from build123d import *

# Parameters (mm, degrees)
F2_DEPTH = 1
F3_W     = 90
F3_H     = 3.5
F3_H_2   = 0.0419686139
F3_H_3   = 3.4580313861
F4_DEPTH = 2
F5_W     = 90
F5_H     = 3.5
F5_H_2   = 4.5
F5_H_3   = 8.0419686139
F6_DEPTH = 1


# Not quite as in the source:
# - a feature names something its author has since deleted; it is built from what else it names


with BuildPart() as f2:
    # F1 (on face) → F2 (new body)
    with BuildSketch(Plane.XY):
        with BuildLine():
            Line((14.8598281033, 4.21106866), (-75.1401718967, 4.21106866))
            Line((-75.1401718967, 4.21106866), (-75.1401718967, 0.21106866))
            Line((-75.1401718967, 0.21106866), (4.3706398308, 0.21106866))
            ThreePointArc((4.3706398308, 0.21106866), (5.7848533932, -0.3747177776), (6.3706398308, -1.78893134))
            Line((6.3706398308, -1.78893134), (6.3706398308, -3.78893134))
            Line((6.3706398308, -3.78893134), (14.8598281033, -3.78893134))
            Line((14.8598281033, -3.78893134), (14.8598281033, 4.21106866))
        make_face()
        with BuildLine():
            Line((14.8598281033, -49.78893134), (6.3706398308, -49.78893134))
            Line((6.3706398308, -49.78893134), (6.3706398308, -51.78893134))
            ThreePointArc((6.3706398308, -51.78893134), (5.7848533932, -53.2031449024), (4.3706398308, -53.78893134))
            Line((4.3706398308, -53.78893134), (-75.1401718967, -53.78893134))
            Line((-75.1401718967, -53.78893134), (-75.1401718967, -57.78893134))
            Line((-75.1401718967, -57.78893134), (14.8598281033, -57.78893134))
            Line((14.8598281033, -57.78893134), (14.8598281033, -49.78893134))
        make_face()
        with BuildLine():
            Line((-75.1401718967, -3.78893134), (-75.1401718967, 0.21106866))
            Line((-75.1401718967, 0.21106866), (-77.6293601692, 0.21106866))
            ThreePointArc((-77.6293601692, 0.21106866), (-79.0435737315, -0.3747177776), (-79.6293601692, -1.78893134))
            Line((-79.6293601692, -1.78893134), (-79.6293601692, -51.78893134))
            ThreePointArc((-79.6293601692, -51.78893134), (-79.0435737315, -53.2031449024), (-77.6293601692, -53.78893134))
            Line((-77.6293601692, -53.78893134), (-75.1401718967, -53.78893134))
            Line((-75.1401718967, -53.78893134), (-75.1401718967, -49.78893134))
            Line((-75.1401718967, -49.78893134), (-75.1401718967, -3.78893134))
        make_face()
        with BuildLine():
            Line((-68.8141618371, -49.78893134), (-75.1401718967, -49.78893134))
            Line((-75.1401718967, -49.78893134), (-75.1401718967, -53.78893134))
            Line((-75.1401718967, -53.78893134), (4.3706398308, -53.78893134))
            ThreePointArc((4.3706398308, -53.78893134), (5.7848533932, -53.2031449024), (6.3706398308, -51.78893134))
            Line((6.3706398308, -51.78893134), (6.3706398308, -49.78893134))
            Line((6.3706398308, -49.78893134), (6.1858381629, -49.78893134))
            Line((6.1858381629, -49.78893134), (0.4592296318, -49.78893134))
            Line((0.4592296318, -49.78893134), (-68.8141618371, -49.78893134))
        make_face()
        with BuildLine():
            Line((4.3706398308, 0.21106866), (-75.1401718967, 0.21106866))
            Line((-75.1401718967, 0.21106866), (-75.1401718967, -3.78893134))
            Line((-75.1401718967, -3.78893134), (-68.8141618371, -3.78893134))
            Line((-68.8141618371, -3.78893134), (6.1858381629, -3.78893134))
            Line((6.1858381629, -3.78893134), (6.3706398308, -3.78893134))
            Line((6.3706398308, -3.78893134), (6.3706398308, -1.78893134))
            ThreePointArc((6.3706398308, -1.78893134), (5.7848533932, -0.3747177776), (4.3706398308, 0.21106866))
        make_face()
    extrude(amount=F2_DEPTH)

    # F3 (on face) → F4 (join)
    with BuildSketch(Plane.XY.offset(1)):
        with Locations((-30.1401718967, 2.46106866)):
            Rectangle(F3_W, F3_H)
        with Locations((-30.1401718967, -57.8099156469)):
            Rectangle(F3_W, F3_H_2)
        with Locations((-30.1401718967, -56.0599156469)):
            Rectangle(F3_W, F3_H_3)
    extrude(amount=F4_DEPTH)

    # F5 (on face) → F6 (join)
    with BuildSketch(Plane.XY.offset(3)):
        with Locations((-30.1401718967, 2.46106866)):
            Rectangle(F5_W, F5_H)
        with Locations((-30.1401718967, -1.53893134)):
            Rectangle(F5_W, F5_H_2)
        with Locations((-30.1401718967, -53.8099156469)):
            Rectangle(F5_W, F5_H_3)
    extrude(amount=F6_DEPTH)


solid = f2.part
The listing builds one solid part. Answer for the finished solid, in the listing's coordinates (mm). A direction names the side the tool comes from. Coordinates: 2 decimals unless noted, no trailing zeros. Loops run counter-clockwise (first coordinate to the right, second up) from the corner with the lowest first, then second, coordinate; pieces in that order, holes last. Notation, with made-up numbers: (27.25, 74) -> (41.25, 74) arc R10 ccw to (41.25, 82) -> close; hole circle Ø6 at (-22.5, 65.25). An arc over 180 degrees is marked (long way). Answer in a Markdown table with one row per item. Add a question column.
1. The part is cut by section C-C, the plane y = -45.5. Write down the section's boundary in (x, z).
2. Flat-ended cylindrical pins translate along their axes: P1, Ø0.5, axis at x = -28, z = 0.5, coming from the -Y side; P2, Ø1.1, axis at x = -76, z = 0.5, coming from the -Y side; P3, Ø0.5, axis at x = -76.5, z = 0.5, coming from the +Y side. Find the tip coordinate at first contact, or state that the pin passes through.
3. Consider line 1 (Y direction, x = -67.5, z = 3.65); line 2 (Y direction, x = -47, z = 2.15); line 3 (Z direction, x = -15.5, y = -50). Determine where each line is inside the solid, lowest interval first. Write a range as [from, to].
4. The part is cut by section B-B, the plane z = 2.2. Write down the section's boundary in (x, y), then the cut area to 3 significant figures.
5. Determine the mould class of faces 5 (the flat face through (-31, -2, 3)), 6 (the flat face through (-31, -54, 4)), 7 (the flat face through (14.86, 1, 2)) for opening direction Z: +Z half, -Z half, draft (parallel to the pull), parting line (faces both ways), or undercut.
6. For faces 1 (the cylindrical face through (-79.03, -0.36, 0.49)), 2 (the flat face through (-40, -51, 1)), 3 (the flat face through (-75.14, 1, 2)), 4 (the flat face through (-75.14, -56, 2)), determine the directions among +Z, -Z, +X, -X, +Y, -Y from which every point of the face is accessible in a straight line to the end or side of a thin tool.
7. The part is cut by section A-A, the plane x = -1. Write down the section's boundary in (y, z).
Answer below:
| question | item | result |
|---|---|---|
| 1 | outline | (-79.63, 0) -> (-75.14, 0) -> (-75.14, 1) -> (-79.63, 1) -> close |
| 2 | P1 | y = -57.79 |
| 2 | P2 | y = -53.79 |
| 2 | P3 | y = 0.21 |
| 3 | line 1 | [-57.83, -49.79], [-3.79, 4.21] |
| 3 | line 2 | [-57.83, -54.33], [0.71, 4.21] |
| 3 | line 3 | [0, 1], [3, 4] |
| 4 | outline | (-75.14, -57.83) -> (14.86, -57.83) -> (14.86, -54.33) -> (-75.14, -54.33) -> close; (-75.14, 0.71) -> (14.86, 0.71) -> (14.86, 4.21) -> (-75.14, 4.21) -> close |
| 4 | area | 630 mm2 |
| 5 | face 5 | undercut |
| 5 | face 6 | +Z half |
| 5 | face 7 | draft |
| 6 | face 1 | +Z, -Z, -X, +Y |
| 6 | face 2 | +X, -X |
| 6 | face 3 | +Z, -X, +Y |
| 6 | face 4 | +Z, -X, -Y |
| 7 | outline | (-57.83, 1) -> (-57.79, 1) -> (-57.79, 0) -> (-49.79, 0) -> (-49.79, 1) -> (-54.33, 1) -> (-54.33, 3) -> (-49.79, 3) -> (-49.79, 4) -> (-57.83, 4) -> close; (-3.79, 0) -> (4.21, 0) -> (4.21, 4) -> (-3.79, 4) -> (-3.79, 3) -> (0.71, 3) -> (0.71, 1) -> (-3.79, 1) -> close |
